Design review of the part shown in the three views and the two pictorial views. Dimensions are in mm from the part's minimum x, y and z. A direction names the side the tool comes from. Round coordinates to 2 decimals unless told otherwise and drop trailing zeros. Write each loop counter-clockwise with the first axis right and the second up, starting at its lowest first coordinate (ties: lowest second). Pieces come first, ordered by that corner, then holes. Notation, with made-up numbers: (19, 39.25) - (63, 39.25) arc R29 ccw to (63, 67.25) - close; hole circle Ø5 at (-37.5, 24). An arc over 180 degrees is marked (long way). Use one line per item in the form item = value.
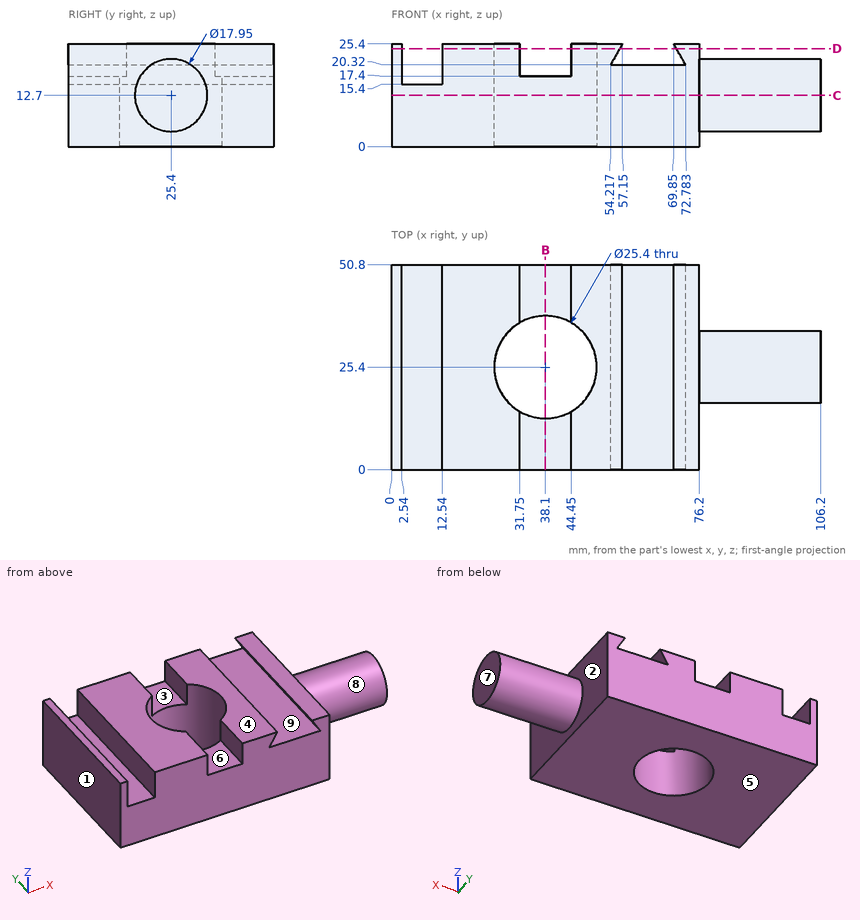
Q1. Machinability: for the marked faces 5, 6, 7, 8 and 9, which of the approach directions +Z, -Z, +X, -X, +Y, -Y give a long, thin tool a straight path to every point of the face, cutting with its end or side? Answer none if there is none.
Calculated:
face_5 = -Z, +X, -X, +Y, -Y
face_6 = +Z, +Y, -Y
face_7 = +Z, -Z, +X, +Y, -Y
face_8 = +X
face_9 = +Y, -Y
Q2. We need section C-C on z = 12.7. Write out the cut boundary in (x, y) (1 decimal), then the cut area to 3 significant figures.
Calculated:
outline = (0, 0) - (76.2, 0) - (76.2, 16.4) - (106.2, 16.4) - (106.2, 34.4) - (76.2, 34.4) - (76.2, 50.8) - (0, 50.8) - close; hole circle Ø25.4 at (38.1, 25.4)
area = 3,900 mm2
Q3. To check wall thickness, follow line 1 along X through (y, z) = (25.4, 18.5); line 2 along X through (y, z) = (26, 14.75); line 3 along Z through (x, y) = (55, 40) (1 decimal). State the ranges of each line that lie inside material, in increasing order. Write a range as from..to.
Calculated:
line_1 = 0..2.54, 12.54..25.4, 50.8..106.2
line_2 = 0..25.41, 50.79..106.2
line_3 = 0..20.3, 21.7..25.4
Q4. For P1, Ø20.5, axis at x = 38.1, y = 25.4, coming from the +Z side; P2, Ø3, axis at y = 35.5, z = 21, coming from the +X side; P3, Ø6, axis at y = 14.5, z = 2.5, coming from the -X side; P4, Ø6.5, axis at x = 40, y = 6, coming from the +Z side, all flat-tipped, find the tip position at first contact; note any pin that passes through.
Calculated:
P1 = through
P2 = 76.2
P3 = 0
P4 = 17.4
Q5. Draft analysis for pull direction X (two halves, no side actions). For the marked faces 1, 2, 3 and 4, state which applies: released by +X, released by -X, zero draft, split by the parting line, or undercut.
Calculated:
face_1 = released by -X
face_2 = released by +X
face_3 = undercut
face_4 = zero draft
Q6. We need section D-D on z = 24.25. Write out the cut boundary in (x, y), then the cut area to 3 significant figures.
Calculated:
outline = (0, 0) - (2.54, 0) - (2.54, 50.8) - (0, 50.8) - close; (12.54, 0) - (31.75, 0) - (31.75, 14.4) arc R12.7 cw to (31.75, 36.4) - (31.75, 50.8) - (12.54, 50.8) - close; (44.45, 0) - (56.49, 0) - (56.49, 50.8) - (44.45, 50.8) - (44.45, 36.4) arc R12.7 cw to (44.45, 14.4) - close; (70.51, 0) - (76.2, 0) - (76.2, 50.8) - (70.51, 50.8) - close
area = 1,810 mm2
Q7. We need section B-B on x = 38.1. Write out the cut boundary in (y, z).
Calculated:
outline = (0, 0) - (12.7, 0) - (12.7, 17.4) - (0, 17.4) - close; (38.1, 0) - (50.8, 0) - (50.8, 17.4) - (38.1, 17.4) - close
